from build123d import *

# Parameters (mm, degrees)
F0_R     = 35
F0_R_2   = 10
F1_DEPTH = 5
F2_R     = 27
F2_R_2   = 10
F3_DEPTH = 15
F0_R_3   = 40
F4_DEPTH = 0.4
F5_R     = 40
F5_R_2   = 36
F6_DEPTH = 4.6
F7_SIZE  = 3.99999


# Not quite as in the source:
# - a fillet or chamfer is up to 0.001 mm smaller than in the source, because OpenCascade refuses the exact size


with BuildPart() as f1:
    # F0 (on Top) → F1 (new body)
    with BuildSketch(Plane.XY):
        Circle(F0_R)
        Circle(F0_R_2, mode=Mode.SUBTRACT)
    extrude(amount=F1_DEPTH)

    # F2 (on face) → F3 (join)
    with BuildSketch(Plane.XY.offset(5)):
        Circle(F2_R)
        Circle(F2_R_2, mode=Mode.SUBTRACT)
    extrude(amount=F3_DEPTH)

    # F0 (on Top) → F4 (join)
    with BuildSketch(Plane.XY):
        Circle(F0_R_3)
        Circle(F0_R, mode=Mode.SUBTRACT)
    extrude(amount=F4_DEPTH)

    # F5 (on face) → F6 (join)
    with BuildSketch(Plane.XY.offset(0.4)):
        Circle(F5_R)
        Circle(F5_R_2, mode=Mode.SUBTRACT)
    extrude(amount=F6_DEPTH)

    # F7 (size 4 in the source; OpenCascade refuses exactly that, so slightly less here)
    f7_edges = [f1.edges().sort_by_distance(p)[0] for p in [
        (-40, 0, 5),
    ]]
    chamfer(f7_edges, length=F7_SIZE)


solid = f1.part
Read the model definition and answer for the solid it produces. Units are mm, in the model's axes. A direction names the side the tool comes from. Give positions to 0.01 mm unless a question says otherwise; leave off trailing zeros. Loops run counter-clockwise (first coordinate to the right, second up) from the corner with the lowest first, then second, coordinate; pieces in that order, holes last. Notation, with made-up numbers: (-38.5, -0.5) -> (20.5, -0.5) arc R11 ccw to (20.5, 11.5) -> close; hole circle Ø2 at (-5.75, -15.75). An arc over 180 degrees is marked (long way). Use a Markdown table: item, result.
Q1. Find the intervals of material crossed by line 1 along X through (y, z) = (-0.5, 14); line 2 along Z through (x, y) = (-18, 26.5); line 3 along Y through (x, z) = (0, 4), in increasing order.
Solved:
| item | result |
|---|---|
| line 1 | x = -27 to -9.99, 9.99 to 27 |
| line 2 | z = 0 to 5 |
| line 3 | y = -37 to -36, -35 to -10, 10 to 35, 36 to 37 |
Q2. A tool of negligible diameter and unlimited length cuts with its end or side. For faces 4 (the face through (-28, -21, 3)), 5 (the face through (12, 0, 20)), from which of +Z, -Z, +X, -X, +Y, -Y can it reach the whole face along a straight path? Write none if from no direction.
Solved:
| item | result |
|---|---|
| face 4 | +Z |
| face 5 | +Z, +X, -X, +Y, -Y |
Q3. Determine the mould class of faces 1 (the face through (-5.85, -26.36, 12.4)), 2 (the face through (8, -8, 0)), 3 (the face through (-2.17, -9.76, 9.86)) for opening direction X: pulls with the +X half, pulls with the -X half, needs draft (parallel to the pull), parting line crosses it, or undercut.
Solved:
| item | result |
|---|---|
| face 1 | parting line crosses it |
| face 2 | needs draft |
| face 3 | undercut |
Q4. Each of these flat-tipped pins is pushed along its axis until it touches: pin 1 (8 mm diameter, centred on x = -22.5, z = 3.5, fed in from -Y); pin 2 (2 mm diameter, centred on y = 14, z = 15, fed in from -X); pin 3 (3 mm diameter, centred on x = -18, z = 13, fed in from +Y). Where does it stop, or does it pass through?
Solved:
| item | result |
|---|---|
| pin 1 | stops at y = -34.99 |
| pin 2 | stops at x = -23.66 |
| pin 3 | stops at y = 21.37 |
Q5. Section C-C, the plane z = 9 is taken. Determine the outline of the cut face in (x, y), then the cut area to 3 significant figures.
Solved:
| item | result |
|---|---|
| outline | circle Ø54 at (0, 0); hole circle Ø20 at (0, 0) |
| area | 1,980 mm^2 |
Q6. Section D-D, the plane z = 3 is taken. Determine the outline of the cut face in (x, y).
Solved:
| item | result |
|---|---|
| outline | circle Ø76 at (0, 0); circle Ø70 at (0, 0); hole circle Ø72 at (0, 0); hole circle Ø20 at (0, 0) |
